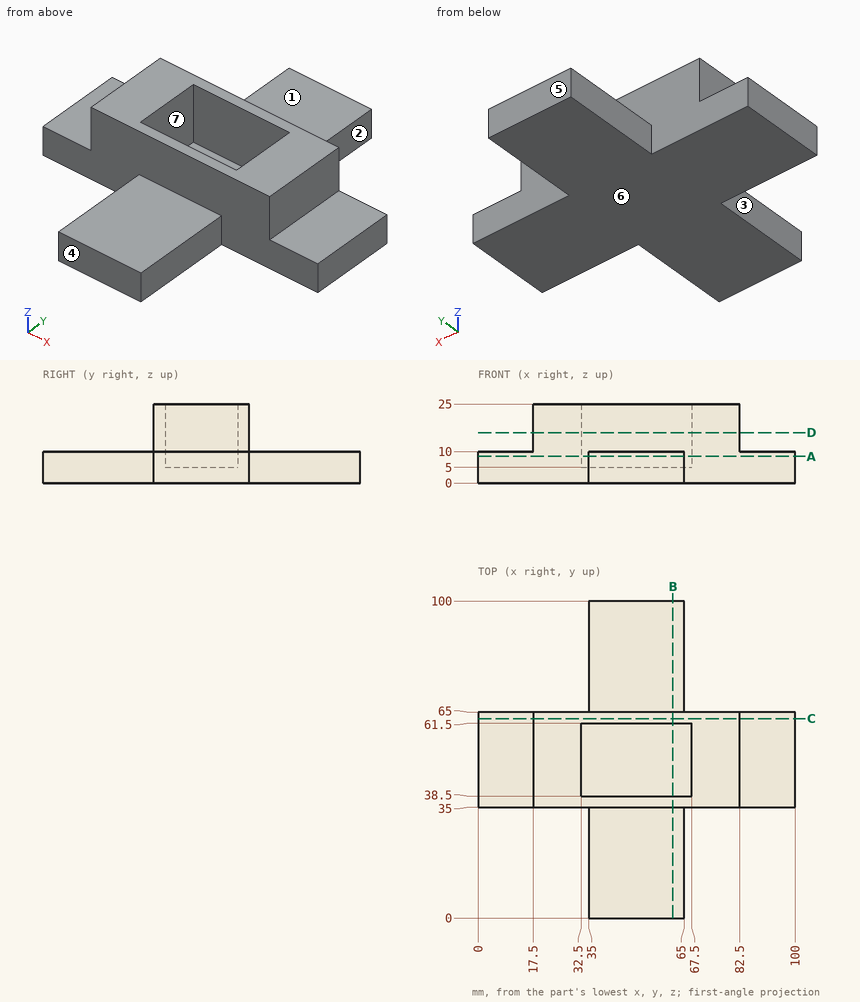
The figure shows three views and two pictorial views of one solid part (mm, origin at its lowest corner). Answer the questions. A direction names the side the tool comes from. Round coordinates to 2 decimals unless told otherwise and drop trailing zeros. Write each loop counter-clockwise with the first axis right and the second up, starting at its lowest first coordinate (ties: lowest second). Pieces come first, ordered by that corner, then holes. Notation, with made-up numbers: (60.5, 8) - (75.5, 8) arc R21 ccw to (75.5, 29) - close; hole circle Ø6 at (83, -37.75). An arc over 180 degrees is marked (long way). Use one line per item in the form item = value. Start each with the question number.
Item 1: Find the intervals of material crossed by line 1 (Y direction, x = 40.5, z = 11.75); line 2 (X direction, y = 50.5, z = 8.75); line 3 (X direction, y = 43, z = 23), in increasing order. Write a range as [from, to].
Item 2: Flat-ended cylindrical pins translate along their axes: pin 1 Ø3 at (y, z) = (37, 12) entering from -X; pin 2 Ø14 at (x, y) = (6, 49.5) entering from +Z; pin 3 Ø1.5 at (x, z) = (18.5, 11) entering from -Y. Find the tip coordinate at first contact, or state that the pin passes through.
Item 3: A cutting plane is placed at C-C (y = 63). Write down the section's boundary in (x, z), plus the area to 4 significant figures.
Item 4: Determine the mould class of the marked faces 4, 5, 6 and 7 for opening direction Y: +Y half, -Y half, draft (parallel to the pull), parting line (faces both ways), or undercut.
Item 5: A cutting plane is placed at D-D (z = 16). Write down the section's boundary in (x, y).
Item 6: A tool of negligible diameter and unlimited length cuts with its end or side. For the marked faces 1, 2 and 3, from which of +Z, -Z, +X, -X, +Y, -Y can it reach the whole face along a straight path? Write none if from no direction.
Item 7: A cutting plane is placed at B-B (x = 61.5). Write down the section's boundary in (y, z), plus the area to 3 significant figures.
Item 8: A cutting plane is placed at A-A (z = 8.5). Write down the section's boundary in (x, y).
The answers:
q1.line_1 = [35, 38.5], [61.5, 65]
q1.line_2 = [0, 32.5], [67.5, 100]
q1.line_3 = [17.5, 32.5], [67.5, 82.5]
q2.pin_1 = 17.5
q2.pin_2 = 10
q2.pin_3 = 35
q3.outline = (0, 0) - (100, 0) - (100, 10) - (82.5, 10) - (82.5, 25) - (17.5, 25) - (17.5, 10) - (0, 10) - close
q3.area = 1,975 mm^2
q4.face_4 = -Y half
q4.face_5 = +Y half
q4.face_6 = draft
q4.face_7 = undercut
q5.outline = (17.5, 35) - (82.5, 35) - (82.5, 65) - (17.5, 65) - close; hole (32.5, 38.5) - (67.5, 38.5) - (67.5, 61.5) - (32.5, 61.5) - close
q6.face_1 = +Z, +X, -X, +Y
q6.face_2 = +Z, -Z, +X, +Y
q6.face_3 = +Z, -Z, -X, -Y
q7.outline = (0, 0) - (100, 0) - (100, 10) - (65, 10) - (65, 25) - (61.5, 25) - (61.5, 5) - (38.5, 5) - (38.5, 25) - (35, 25) - (35, 10) - (0, 10) - close
q7.area = 990 mm^2
q8.outline = (0, 35) - (35, 35) - (35, 0) - (65, 0) - (65, 35) - (100, 35) - (100, 65) - (65, 65) - (65, 100) - (35, 100) - (35, 65) - (0, 65) - close; hole (32.5, 38.5) - (67.5, 38.5) - (67.5, 61.5) - (32.5, 61.5) - close
